For this review, use the dimensioned drawing (mm, ordinates from the lowest corner) and the shaded views. A direction names the side the tool comes from. Round coordinates to 2 decimals unless told otherwise and drop trailing zeros. Loops run counter-clockwise (first coordinate to the right, second up) from the corner with the lowest first, then second, coordinate; pieces in that order, holes last. Notation, with made-up numbers: (82.5, -2) - (133.5, -2) arc R13 ccw to (133.5, 9) - close; hole circle Ø3 at (-4, -32). An arc over 180 degrees is marked (long way). Use one line per item in the form item = value. Start each with the question number.
(1) We need section C-C, the plane x = 22. Write out the cut boundary in (y, z) (1 decimal).
(2) We need section A-A, the plane y = 10.5. Write out the cut boundary in (x, z) (1 decimal).
(3) Wall thickness on probe 1 along X at (y, z) = (22, 1); probe 2 along Y at (x, z) = (30, 8.25) (1 decimal); probe 3 along Z at (x, y) = (21, 15) (1 decimal): over which ranges is each line inside the solid? List them lowest first. Write a range as [from, to].
(4) We need section B-B, the plane z = 9.25. Give the number of separate pieces and of enclosed holes in the cut face, then the cut area to 3 significant figures.
(5) Machinability: for the marked faces 4, 5 and 6, which of the approach directions +Z, -Z, +X, -X, +Y, -Y give a long, thin tool a straight path to every point of the face, cutting with its end or side? Answer none if there is none.
(6) For pin 1 (8 mm diameter, centred on x = 50.5, y = 7, fed in from +Z); pin 2 (7.5 mm diameter, centred on x = 44, z = 10, fed in from +Y) (1 decimal); pin 3 (5 mm diameter, centred on y = 14, z = 11.5, fed in from +X), all flat-tipped, find the tip position at first contact; note any pin that passes through.
(7) The part is to be moulded in two halves that separate along Z. For the marked faces 1, 2 and 3, say which applies: released by +Z, released by -Z, zero draft, split by the parting line, or undercut.
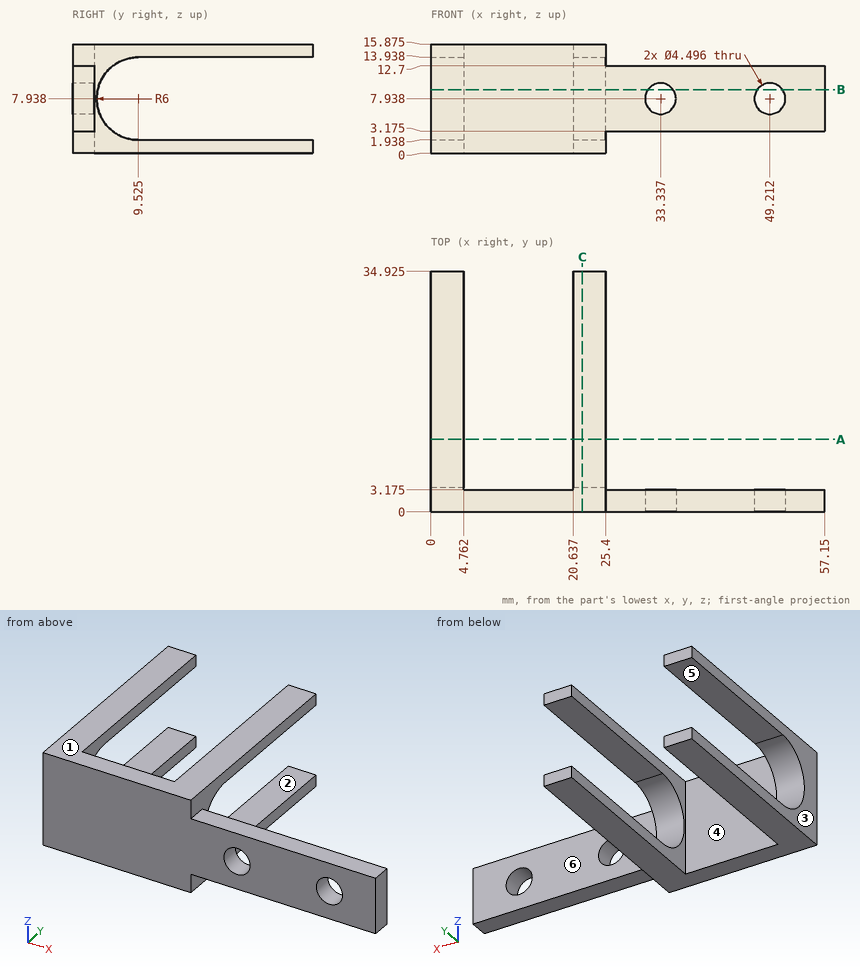
Data:
q1.outline = (0, 0) - (34.9, 0) - (34.9, 1.9) - (9.5, 1.9) arc R6 cw to (9.5, 13.9) - (34.9, 13.9) - (34.9, 15.9) - (0, 15.9) - close
q2.outline = (0, 0) - (4.8, 0) - (4.8, 1.9) - (0, 1.9) - close; (0, 13.9) - (4.8, 13.9) - (4.8, 15.9) - (0, 15.9) - close; (20.6, 0) - (25.4, 0) - (25.4, 1.9) - (20.6, 1.9) - close; (20.6, 13.9) - (25.4, 13.9) - (25.4, 15.9) - (20.6, 15.9) - close
q3.probe_1 = [0, 4.76], [20.64, 25.4]
q3.probe_2 = [0, 3.2]
q3.probe_3 = [0, 1.9], [13.9, 15.9]
q4.separate_pieces = 3
q4.enclosed_holes = 0
q4.area = 163 mm^2
q5.face_4 = +Z, -Z, +Y
q5.face_5 = +X, -X, +Y
q5.face_6 = +Z, -Z, +X, +Y
q6.pin_1 = 12.7
q6.pin_2 = 3.2
q6.pin_3 = 25.4
q7.face_1 = released by +Z
q7.face_2 = undercut
q7.face_3 = zero draft
